Study the drawing (mm; zero at the part's minimum x, y, z) and answer. Coordinates: 2 decimals unless noted, no trailing zeros. Loops run counter-clockwise (first coordinate to the right, second up) from the corner with the lowest first, then second, coordinate; pieces in that order, holes last. Notation, with made-up numbers: (48, -11) - (65, -11) arc R21 ccw to (65, 25) - close; hole circle Ø3 at (61.5, 41). An arc over 180 degrees is marked (long way). Put each result on its own line as item: value.
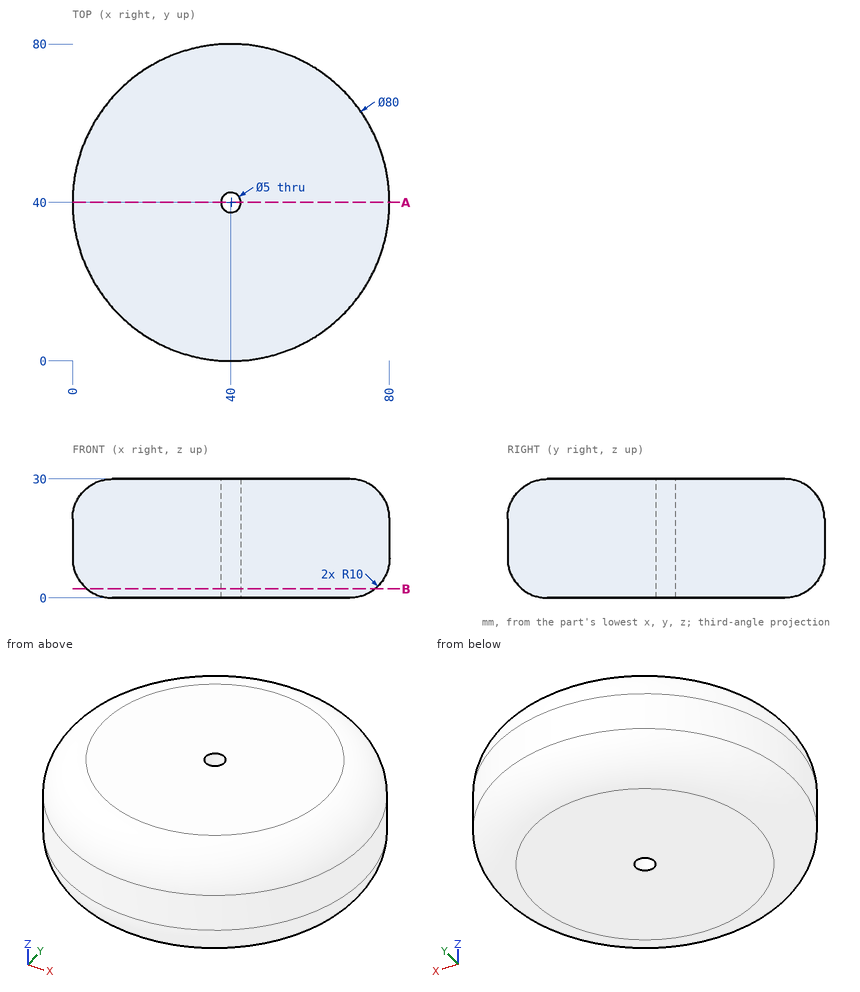
1) Each of these flat-tipped pins is pushed along its axis until it touches: pin 1 (8 mm diameter, centred on y = 15.5, z = 19.5, fed in from -X); pin 2 (4 mm diameter, centred on y = 70.5, z = 3.5, fed in from -X); pin 3 (6 mm diameter, centred on y = 14, z = 14.5, fed in from -X). Where does it stop, or does it pass through?
Found:
pin 1: stops at x = 5.65
pin 2: stops at x = 14.59
pin 3: stops at x = 7.27
2) The part is cut by section B-B (z = 2.25). Give the vertices of the cut face in (x, y).
Found:
outline: circle Ø72.64 at (40, 40); hole circle Ø5 at (40, 40)
3) The part is cut by section A-A (y = 40). Give the vertices of the cut face in (x, z), and give its area (3 significant figures).
Found:
outline: (0, 10) arc R10 ccw to (10, 0) - (37.5, 0) - (37.5, 30) - (10, 30) arc R10 ccw to (0, 20) - close; (42.5, 0) - (70, 0) arc R10 ccw to (80, 10) - (80, 20) arc R10 ccw to (70, 30) - (42.5, 30) - close
area: 2,160 mm^2
4) Straight lines are drawn through the part: L1, parallel to Y at x = 40, z = 20; L2, parallel to Y at x = 40, z = 24.25; L3, parallel to Z at x = 25.5, y = 69. For each, find the intervals that lie inside material, in ascending order. Write a range as [from, to].
Found:
L1: y = [0, 37.5], [42.5, 80]
L2: y = [0.95, 37.5], [42.5, 79.05]
L3: z = [0.3, 29.7]
